Check sheet for the modelled part. Datum: model origin and axes. Units: mm. A direction names the side the tool comes from. Round coordinates to 2 decimals unless told otherwise and drop trailing zeros. Write each loop counter-clockwise with the first axis right and the second up, starting at its lowest first coordinate (ties: lowest second). Pieces come first, ordered by that corner, then holes.
Autodesk Inventor part; units mm, degrees
ref_plane "YZ Plane" through (0, 0, 0) normal (1, 0, 0) x (0, 1, 0)
ref_plane "XZ Plane" through (0, 0, 0) normal (0, 1, 0) x (-1, 0, 0)
ref_plane "XY Plane" through (0, 0, 0) normal (0, 0, 1) x (1, 0, 0)
sketch "Sketch1" plane through (0, 0, 0) normal (0, 1, 0) x (-1, 0, 0)
  line L0 (-384.175, -384.175) -> (384.175, -384.175)
  line L1 (384.175, -384.175) -> (384.175, 384.175)
  line L2 (384.175, 384.175) -> (-384.175, 384.175)
  line L3 (-384.175, 384.175) -> (-384.175, -384.175)
  line L4 (-384.175, -384.175) -> (384.175, 384.175) construction
  line L5 (384.175, -384.175) -> (-384.175, 384.175) construction
  line L6 (441.325, 441.325) -> (441.325, -441.325)
  line L7 (441.325, -441.325) -> (-441.325, -441.325)
  line L8 (-441.325, -441.325) -> (-441.325, 441.325)
  line L9 (-441.325, 441.325) -> (441.325, 441.325)
  point P0 (0, 0)
  dimension "d0" = 768.35
  dimension "d1" = 768.35
  dimension "d2" = 57.15
extrude "Extrusion1" add sketch "Sketch1" along normal blind 127
fillet "Fillet1" radius 38.1 4 edges at (-441.325, 63.5, 441.325) (441.325, 63.5, 441.325) (441.325, 63.5, -441.325) (-441.325, 63.5, -441.325)
fillet "Fillet2" radius 25.4 16 edges at (430.1658, 127, 430.1658) (441.325, 127, 0) (430.1658, 127, -430.1658) (0, 127, -441.325) (-430.1658, 127, -430.1658) (-441.325, 127, 0) (-430.1658, 127, 430.1658) (0, 127, 441.325) (430.1658, 0, 430.1658) (441.325, 0, 0) (430.1658, 0, -430.1658) (0, 0, -441.325) (-430.1658, 0, -430.1658) (-441.325, 0, 0) (-430.1658, 0, 430.1658) (0, 0, 441.325)
properties part number "BP-0036" material "Fabric"
1. Release check for a two-part mould opening along Z. For faces 1 (the cylindrical face through (5.645, 7.243, -433.687)), 2 (the cylindrical face through (429.87, 64.03, 430.46)), 3 (the flat face through (-384.175, 63, -5)) record: released by +Z, released by -Z, zero draft, split by the parting line, or undercut.
2. Set-up check for faces 4 (the cylindrical face through (-430.46, 64.03, 429.87)), 5 (the flat face through (5, 63, -384.175)): record each of +Z, -Z, +X, -X, +Y, -Y from which the full face is reachable in a straight line by a thin tool's end or side.
3. Sectioned sample at B-B, the plane z = 291. Enter the section's corners in (x, y) (3 decimals).
4. Sectioned sample at C-C, the plane y = 61. Enter the section's corners in (x, z) (3 decimals).
5. Go/stop test with a flat-tipped pin: pin 1 (10 mm diameter, centred on y = 15, z = -228.5, fed in from -X). Record where the tip stops, or that it passes through.
6. Sectioned sample at A-A, the plane x = 260. Enter the section's corners in (y, z) (3 decimals), plus the area to 3 significant figures.
7. Scan lines: line 1 along Z through (x, y) = (160.5, 100) (3 decimals); line 2 along Z through (x, y) = (145.5, 13.5) (3 decimals). Record each from-to range of solid material in increasing order.
Computed values:
1. face 1: released by -Z
1. face 2: released by +Z
1. face 3: undercut
2. face 4: +Z, -X, +Y, -Y
2. face 5: +Y, -Y
3. outline: (-441.325, 25.4) arc R25.4 ccw to (-415.925, 0) - (-384.175, 0) - (-384.175, 127) - (-415.925, 127) arc R25.4 ccw to (-441.325, 101.6) - close; (384.175, 0) - (415.925, 0) arc R25.4 ccw to (441.325, 25.4) - (441.325, 101.6) arc R25.4 ccw to (415.925, 127) - (384.175, 127) - close
4. outline: (-441.325, -403.225) arc R38.1 ccw to (-403.225, -441.325) - (403.225, -441.325) arc R38.1 ccw to (441.325, -403.225) - (441.325, 403.225) arc R38.1 ccw to (403.225, 441.325) - (-403.225, 441.325) arc R38.1 ccw to (-441.325, 403.225) - close; hole (-384.175, -384.175) - (384.175, -384.175) - (384.175, 384.175) - (-384.175, 384.175) - close
5. pin 1: stops at x = -440.74
6. outline: (0, -415.925) arc R25.4 ccw to (25.4, -441.325) - (101.6, -441.325) arc R25.4 ccw to (127, -415.925) - (127, -384.175) - (0, -384.175) - close; (0, 384.175) - (127, 384.175) - (127, 415.925) arc R25.4 ccw to (101.6, 441.325) - (25.4, 441.325) arc R25.4 ccw to (0, 415.925) - close
6. area: 14,000 mm2
7. line 1: z = -441.325 to -384.175, 384.175 to 441.325
7. line 2: z = -438.365 to -384.175, 384.175 to 438.365
